Here's how the part is built. I have some questions about the finished solid (model axes, mm). A direction names the side the tool comes from. Coordinates: 2 decimals unless noted, no trailing zeros. Order: outer loops, then holes, each group sorted by start corner. A loop starts at its lowest first (then second) coordinate and runs counter-clockwise, first axis right, second up. Notation, with made-up numbers: (-31.75, 24.25) - (-27.75, 24.25) arc R20 cw to (-27.75, 31.25) - close; hole circle Ø9 at (-22.5, 15.25). An arc over 180 degrees is marked (long way). Answer in a Markdown table with one row per item. Add a question column.
Item 1: On a 3-axis mill with a long thin cutter (end or side, diameter ignored), from which of +Z, -Z, +X, -X, +Y, -Y can I reach the whole of each face in a straight line? I mean faces 4 (the flat face through (-3, -55, 9)), 5 (the flat face through (-2, -99, -20.271)). Say none if no direction works.
Item 2: Thinking about a two-plate mould opening in Y: for faces 1 (the cylindrical face through (-3, -116, 0)), 2 (the cylindrical face through (-2.08, -3.01, -17.42)), 3 (the cylindrical face through (-3.29, -197.15, 26.72)), which applies, +Y half, -Y half, draft (parallel to the pull), parting line (faces both ways), or undercut?
Item 3: Will these pins go through, and if not, where does the flat tip stop? pin 1 Ø5 at (y, z) = (-66.5, 10) entering from -X; pin 2 Ø12 at (y, z) = (-31.5, -6) entering from -X; pin 3 Ø1 at (y, z) = (-27.5, 15) entering from -X.
Item 4: If I drill on line 1 along Z through (x, y) = (-6, -36); line 2 along Y through (x, z) = (-9.75, -6); line 3 along Y through (x, z) = (-7.75, -2), over which ranges is the centre line in solid material (lowest first)? Write a range as from..to.
Item 5: I want a section at A-A (z = -7). Please give me the cut outline in (x, y).
Item 6: I want a section at B-B (x = -8). Please give me the cut outline in (y, z).
Item 7: I want a section at D-D (z = 23). Please give me the cut outline in (x, y).
Item 8: I want a section at C-C (y = -91). Please give me the cut outline in (x, z).
```python
from build123d import *

# Parameters (mm, degrees)
F1_DEPTH = 200
F3_DEPTH = 20.001
F4_R     = 10


with BuildPart() as f1:
    # F0 (on Front) → F1 (new body)
    with BuildSketch(Plane.XZ):
        Polygon((6.850831, -20.271453), (6.850831, 29.728547), (-13.149169, 29.728547), (-10.791229, -20.271453), align=None)
    extrude(amount=F1_DEPTH)

    # F2 (on face) → F3 (cut, through all)
    with BuildSketch(Plane.YZ.offset(6.850831)):
        with BuildLine():
            Line((-125, 9), (-165, 9))
            ThreePointArc((-165, 9), (-174, 0), (-165, -9))
            Line((-165, -9), (-125, -9))
            ThreePointArc((-125, -9), (-116, 0), (-125, 9))
        make_face()
        with BuildLine():
            Line((-35, 9), (-75, 9))
            ThreePointArc((-75, 9), (-84, 0), (-75, -9))
            Line((-75, -9), (-35, -9))
            ThreePointArc((-35, -9), (-26, 0), (-35, 9))
        make_face()
    extrude(amount=-F3_DEPTH, mode=Mode.SUBTRACT)

    # F4
    f4_edges = [f1.edges().sort_by_distance(p)[0] for p in [
        (-3.149169, -200, 29.728547),
        (-1.970199, -200, -20.271453),
        (-1.970199, 0, -20.271453),
        (-3.149169, 0, 29.728547),
    ]]
    fillet(f4_edges, radius=F4_R)


solid = f1.part
```
Values follow:
| question | item | result |
|---|---|---|
| 1 | face 4 | +X, -X |
| 1 | face 5 | -Z, +X, -X, +Y, -Y |
| 2 | face 1 | undercut |
| 2 | face 2 | +Y half |
| 2 | face 3 | -Y half |
| 3 | pin 1 | stops at x = -12.34 |
| 3 | pin 2 | stops at x = -11.62 |
| 3 | pin 3 | stops at x = -12.48 |
| 4 | line 1 | z = -20.27..-9, 9..29.73 |
| 4 | line 2 | y = -200..-171.71, -118.29..-81.71, -28.29..0 |
| 4 | line 3 | y = -200..-173.77, -116.23..-83.77, -26.23..0 |
| 5 | outline | (-11.42, -200) - (6.85, -200) - (6.85, -170.66) - (-11.42, -170.66) - close; (-11.42, -119.34) - (6.85, -119.34) - (6.85, -80.66) - (-11.42, -80.66) - close; (-11.42, -29.34) - (6.85, -29.34) - (6.85, 0) - (-11.42, 0) - close |
| 6 | outline | (-200, -10.27) arc R10 ccw to (-190, -20.27) - (-10, -20.27) arc R10 ccw to (0, -10.27) - (0, 19.73) arc R10 ccw to (-10, 29.73) - (-190, 29.73) arc R10 ccw to (-200, 19.73) - close; hole (-165, -9) - (-125, -9) arc R9 ccw to (-125, 9) - (-165, 9) arc R9 ccw to start; hole (-75, -9) - (-35, -9) arc R9 ccw to (-35, 9) - (-75, 9) arc R9 ccw to start |
| 7 | outline | (-12.83, -199.45) - (6.85, -199.45) - (6.85, -0.55) - (-12.83, -0.55) - close |
| 8 | outline | (-13.15, 29.73) - (-10.79, -20.27) - (6.85, -20.27) - (6.85, 29.73) - close |
